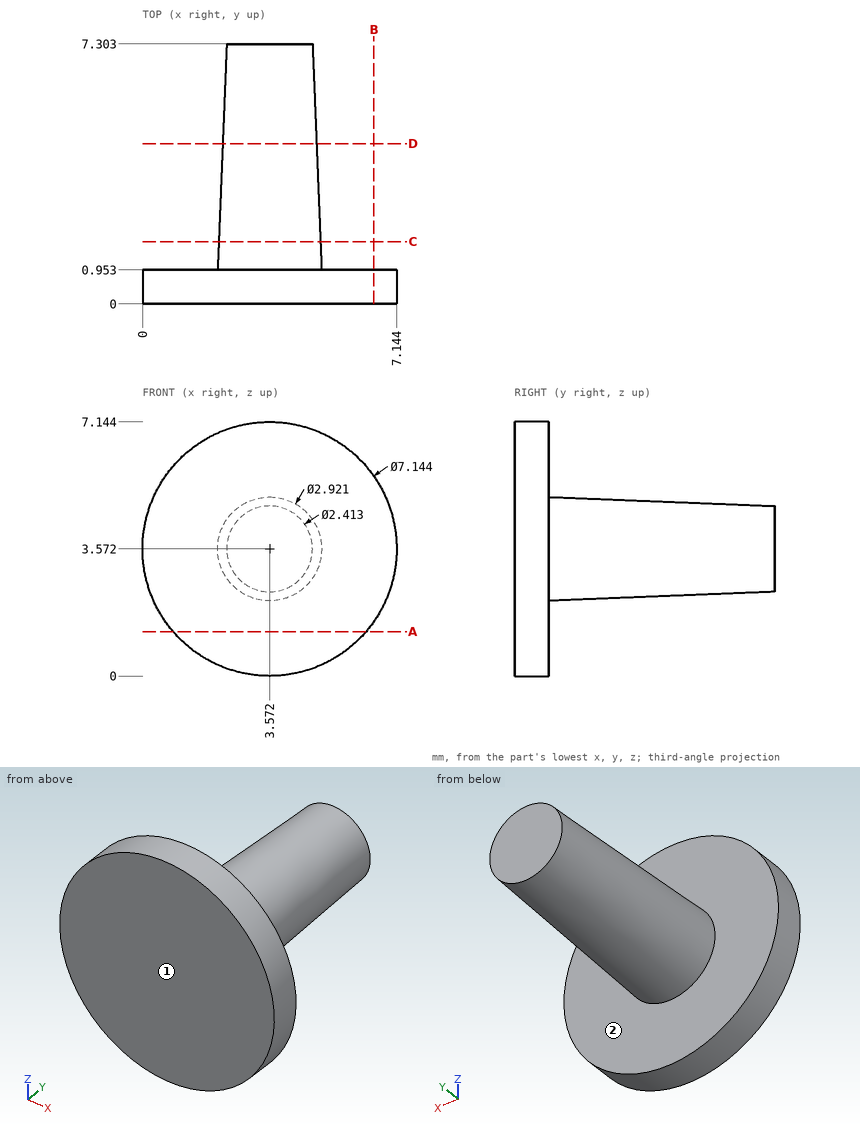
Geometry check sheet. Reference: drawing and pictorial views, mm from the part's lowest x, y, z. A direction names the side the tool comes from. Give positions to 0.01 mm unless a question says otherwise; leave off trailing zeros. Write each loop counter-clockwise with the first axis right and the second up, starting at its lowest first coordinate (ties: lowest second). Pieces come first, ordered by that corner, then holes.
Item 1: Gauge pin test, flat ends, axial feed: pin 1 (2 mm diameter, centred on x = 1.5, y = 4.5, fed in from +Z); pin 2 (3 mm diameter, centred on y = 3, z = 3.5, fed in from -X). Record the tip position at first contact, or that the pin passes through.
Item 2: Access from +Z, -Z, +X, -X, +Y, -Y to the whole of each face (thin tool, end or side, straight path). Record for the marked faces 1 and 2.
Item 3: Cross-section at C-C (y = 1.75). Enter the section's corners in (x, z).
Item 4: Scan lines: L1, parallel to X at y = 5.5, z = 4 (1 decimal); L2, parallel to Y at x = 2.5, z = 6.5; L3, parallel to X at y = 3.75, z = 3.25. Record each from-to range of solid material in increasing order.
Item 5: Cross-section at B-B (x = 6.5). Enter the section's corners in (y, z).
Item 6: Cross-section at D-D (y = 4.5). Enter the section's corners in (x, z).
Item 7: Cross-section at A-A (z = 1.25). Enter the section's corners in (x, y).
Report:
1. pin 1: stops at z = 4.34
1. pin 2: stops at x = 2.13
2. face 1: +Z, -Z, +X, -X, -Y
2. face 2: +Y
3. outline: circle Ø2.86 at (3.57, 3.57)
4. L1: x = 2.4 to 4.8
4. L2: y = 0 to 0.95
4. L3: x = 2.26 to 4.88
5. outline: (0, 1.53) - (0.95, 1.53) - (0.95, 5.62) - (0, 5.62) - close
6. outline: circle Ø2.64 at (3.57, 3.57)
7. outline: (0.86, 0) - (6.29, 0) - (6.29, 0.95) - (0.86, 0.95) - close
